The model under review builds one solid part; all positions refer to its coordinate system, in mm. A direction names the side the tool comes from. Coordinates: 2 decimals unless noted, no trailing zeros. Write each loop counter-clockwise with the first axis right and the second up, starting at its lowest first coordinate (ties: lowest second). Pieces come first, ordered by that corner, then holes.
```python
from build123d import *
from build123d.topology import SkipClean

# Parameters (mm, degrees)
BASISVLAK_W          = 60
BASISVLAK_H          = 60
BASIS_DEPTH          = 5
CIRKELS_HOUDER_R     = 12
CIRKELS_HOUDER_R_2   = 10
HOUDER_DEPTH         = 40
CIRKEL_GAT_R         = 2
GATEN_DEPTH          = 59.309518948
GAT_KABELS_REACH     = 63.847
CIRKEL_GAT_KABELS_R  = 2.5
RIBBE_START          = -2
RIBBE_DEPTH          = 4
RIBBEN_PATROON_COUNT = 4
GLEUF_REACH          = 82.777
GLEUF_END_RADIUS     = 2.5
VIERKANT_BASIS_W     = 2.5
VIERKANT_BASIS_H     = 3


# Read off the part's stored shape, not the designer's step: Ribbe
with BuildPart() as part:
    # Basisvlak → Basis (new body)
    with BuildSketch(Plane(origin=(0, 0, 0), x_dir=(1, 0, 0), z_dir=(0, 1, 0))):
        Rectangle(BASISVLAK_W, BASISVLAK_H)
    extrude(amount=BASIS_DEPTH)

    # Cirkels houder → Houder (add)
    with BuildSketch(Plane(origin=(0, 5, 0), x_dir=(1, 0, 0), z_dir=(0, 1, 0))):
        with Locations(Location((0, 0, 0), (0, 0, 90))):
            Circle(CIRKELS_HOUDER_R)
        with Locations(Location((0, 0, 0), (0, 0, 270))):
            Circle(CIRKELS_HOUDER_R_2, mode=Mode.SUBTRACT)
    extrude(amount=HOUDER_DEPTH)

    # Cirkel gat → Gaten (cut, through all)
    with BuildSketch(Plane(origin=(0, 5, 0), x_dir=(1, 0, 0), z_dir=(0, 1, 0))):
        with Locations(Location((-20, -20, 0), (0, 0, 270))):
            Circle(CIRKEL_GAT_R)
        with Locations(Location((20, -20, 0), (0, 0, 270))):
            Circle(CIRKEL_GAT_R)
        with Locations(Location((-20, 20, 0), (0, 0, 270))):
            Circle(CIRKEL_GAT_R)
        with Locations(Location((20, 20, 0), (0, 0, 270))):
            Circle(CIRKEL_GAT_R)
    extrude(amount=-GATEN_DEPTH, mode=Mode.SUBTRACT)

    # Cirkel gat kabels → Gat kabels (cut, up to next)
    with BuildSketch(Plane(origin=(0, 0, 0), x_dir=(-1, 0, 0), z_dir=(0, -1, 0)), mode=Mode.PRIVATE) as gat_kabels_sk1:
        with Locations(Location((0, 0, 0), (0, 0, 90))):
            Circle(CIRKEL_GAT_KABELS_R)
    gat_kabels_tool1 = extrude(gat_kabels_sk1.sketch, amount=-GAT_KABELS_REACH, mode=Mode.PRIVATE) & part.part
    add(gat_kabels_tool1.solids().sort_by_distance((0, 0, 0))[0], mode=Mode.SUBTRACT)

    # Ribbe outline → Ribbe (add)
    with BuildSketch(Plane(origin=(0, 0, 0), x_dir=(0, 0, -1), z_dir=(1, 0, 0)).offset(RIBBE_START)):
        Polygon((30, 5), (11, 43), (10, 43), (10, 5), align=None)
    ribbe = extrude(amount=RIBBE_DEPTH)

    # Ribben patroon: Ribbe ×4 about axis
    with SkipClean():  # the faces are left unmerged after this step: merging them gives an invalid solid
        ribben_patroon_axis = Axis((0, 0, 0), (0, 1, 0))
        for i in range(1, RIBBEN_PATROON_COUNT):
            add(ribbe.rotate(ribben_patroon_axis, i * 360 / RIBBEN_PATROON_COUNT))

    # Gleuf: up to this cylinder (the profile starts outside it)
    with SkipClean():  # the faces are left unmerged after this step: merging them gives an invalid solid
        gleuf_end = Plane(origin=(0, 1.5, 0), z_dir=(0, -1, 0)) * Cylinder(GLEUF_END_RADIUS, 171.554, mode=Mode.PRIVATE)
        # vierkant_basis → Gleuf (cut, up to the surface)
        with BuildSketch(Plane.XY.offset(30), mode=Mode.PRIVATE) as gleuf_sk1:
            with Locations((0, 1.5)):
                Rectangle(VIERKANT_BASIS_W, VIERKANT_BASIS_H)
        gleuf_tool1 = extrude(gleuf_sk1.sketch, amount=-GLEUF_REACH, mode=Mode.PRIVATE) - gleuf_end
        add(gleuf_tool1.solids().sort_by_distance((0, 1.5, 30))[0], mode=Mode.SUBTRACT)


solid = part.part
```
Item 1: Take a section at B-B, the plane z = 20. Write out the cut boundary in (x, y), plus the area to 4 significant figures.
Solved:
outline: (-30, 0) - (-22, 0) - (-22, 5) - (-30, 5) - close; (-18, 0) - (-1.25, 0) - (-1.25, 3) - (1.25, 3) - (1.25, 0) - (18, 0) - (18, 5) - (2, 5) - (2, 25) - (-2, 25) - (-2, 5) - (-18, 5) - close; (22, 0) - (30, 0) - (30, 5) - (22, 5) - close
area: 332.5 mm2
Item 2: Mouldability with a two-part tool opening along Z and no side actions: class faces 1 (the face through (0, 3, 16)), 2 (the face through (17, 15, -2)), 3 (the face through (0.751, 2.465, -2.385)) as pulls with the +Z half, pulls with the -Z half, needs draft (parallel to the pull), parting line crosses it, or undercut.
Solved:
face 1: needs draft
face 2: pulls with the -Z half
face 3: undercut
Item 3: Take a section at D-D, the plane x = 0. Write out the cut boundary in (y, z), plus the area to 3 significant figures.
Solved:
outline: (0, -30) - (5, -30) - (41, -12) - (45, -12) - (45, -10) - (5, -10) - (5, -2.5) - (0, -2.5) - close; (3, 2.5) - (5, 2.5) - (5, 10) - (45, 10) - (45, 12) - (41, 12) - (5, 30) - (3, 30) - close
area: 1,000 mm2
Item 4: For pin 1 (8 mm diameter, centred on x = -10, z = -18.5, fed in from +Y); pin 2 (4 mm diameter, centred on x = 0, y = 16.5, fed in from -Z); pin 3 (1.5 mm diameter, centred on y = 8, z = 19.5, fed in from +X), all flat-tipped, find the tip position at first contact; note any pin that passes through.
Solved:
pin 1: stops at y = 5
pin 2: stops at z = -25.25
pin 3: stops at x = 2
Item 5: Take a section at A-A, the plane x = 20. Write out the cut boundary in (y, z), plus the area to 3 significant figures.
Solved:
outline: (0, -30) - (5, -30) - (5, -22) - (0, -22) - close; (0, -18) - (5, -18) - (5, -2) - (25, -2) - (25, 2) - (5, 2) - (5, 18) - (0, 18) - close; (0, 22) - (5, 22) - (5, 30) - (0, 30) - close
area: 340 mm2
Item 6: Take a section at C-C, the plane y = 26.5. Write out the cut boundary in (x, z).
Solved:
outline: (-19.25, -2) - (-11.83, -2) arc R12 ccw to (-2, -11.83) - (-2, -19.25) - (2, -19.25) - (2, -11.83) arc R12 ccw to (11.83, -2) - (19.25, -2) - (19.25, 2) - (11.83, 2) arc R12 ccw to (2, 11.83) - (2, 19.25) - (-2, 19.25) - (-2, 11.83) arc R12 ccw to (-11.83, 2) - (-19.25, 2) - close; hole circle Ø20 at (0, 0)
Item 7: Machinability: for faces 4 (the face through (16, 5, -16)), 5 (the face through (2, 15, 17)), 6 (the face through (-17, 15, 2)), which of the approach directions +Z, -Z, +X, -X, +Y, -Y give a long, thin tool a straight path to every point of the face, cutting with its end or side? Answer none if there is none.
Solved:
face 4: -Z, +X, +Y
face 5: +Z, +X, +Y
face 6: +Z, -X, +Y
Item 8: To check wall thickness, follow line 1 along X through (y, z) = (1.55, 20); line 2 along X through (y, z) = (2, -20); line 3 along Z through (x, y) = (-0.5, 41.5). State the ranges of each line that lie inside material, in increasing order.
Solved:
line 1: x = -30 to -22, -18 to -1.25, 1.25 to 18, 22 to 30
line 2: x = -30 to -22, -18 to 18, 22 to 30
line 3: z = -11.99 to -9.99, 9.99 to 11.99
